Model file for the job. Use its own axes, mm. Round coordinates to 2 decimals unless told otherwise and drop trailing zeros. Write each loop counter-clockwise with the first axis right and the second up, starting at its lowest first coordinate (ties: lowest second). Pieces come first, ordered by that corner, then holes. Notation, with made-up numbers: (-10, 7) - (36, 7) arc R30 ccw to (36, 32) - close; hole circle Ø4 at (-11.5, 71). An arc over 180 degrees is marked (long way). Answer as a JSON object with one key per item and string values. Group by question number.
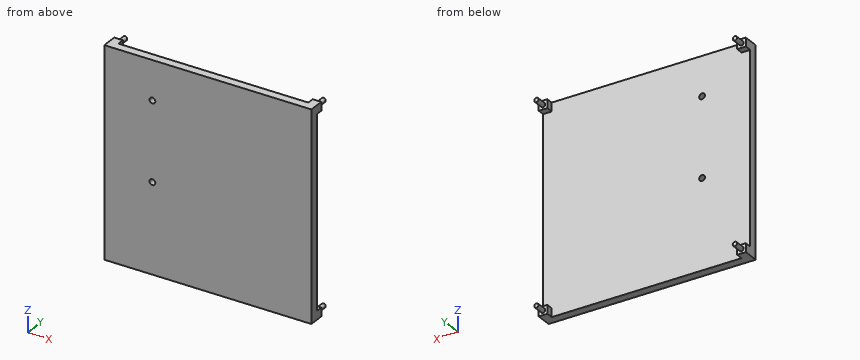
from build123d import *

# Parameters (mm, degrees)
STOCK_PLATE_BETA1_1_OUTLINE_W   = 152.4
STOCK_PLATE_BETA1_1_OUTLINE_H   = 152.4
STOCK_PLATE_BETA1_1_OUTLINE_R   = 2.125
STOCK_PLATE_BETA1_1_DEPTH       = 6.35
STOCK_PLATE_BETA1_1_START       = 6.35
STOCK_PLATE_BETA1_1_2_OUTLINE_W = 6.35
STOCK_PLATE_BETA1_1_2_OUTLINE_H = 6.35
STOCK_PLATE_BETA1_1_2_DEPTH     = 5.08
SKETCH1_R                       = 1.5875
BOSS_EXTRUDE1_DEPTH             = 7.62


# Read off the part's stored shape, not the designer's step: Stock-plate_beta1-1
with BuildPart() as part:
    # Stock-plate_beta1-1 outline → Stock-plate_beta1-1 (new body)
    with BuildSketch(Plane(origin=(0, 0, 0), x_dir=(1, 0, 0), z_dir=(0, 1, 0))):
        with Locations((40.776583963, 45.362139437)):
            Rectangle(STOCK_PLATE_BETA1_1_OUTLINE_W, STOCK_PLATE_BETA1_1_OUTLINE_H)
        with Locations((0, -2.125)):
            Circle(STOCK_PLATE_BETA1_1_OUTLINE_R, mode=Mode.SUBTRACT)
        with Locations((0, 55.889)):
            Circle(STOCK_PLATE_BETA1_1_OUTLINE_R, mode=Mode.SUBTRACT)
    extrude(amount=STOCK_PLATE_BETA1_1_DEPTH)

    # Stock-plate_beta1-1 2 outline → Stock-plate_beta1-1 2 (add)
    with BuildSketch(Plane(origin=(0, 0, 0), x_dir=(1, 0, 0), z_dir=(0, 1, 0)).offset(STOCK_PLATE_BETA1_1_START)):
        with Locations((113.801583963, 118.387139437)):
            Rectangle(STOCK_PLATE_BETA1_1_2_OUTLINE_W, STOCK_PLATE_BETA1_1_2_OUTLINE_H)
        with Locations((-32.248416037, 118.387139437)):
            Rectangle(STOCK_PLATE_BETA1_1_2_OUTLINE_W, STOCK_PLATE_BETA1_1_2_OUTLINE_H)
        with Locations((113.801583963, -27.662860563)):
            Rectangle(STOCK_PLATE_BETA1_1_2_OUTLINE_W, STOCK_PLATE_BETA1_1_2_OUTLINE_H)
        with Locations((-32.248416037, -27.662860563)):
            Rectangle(STOCK_PLATE_BETA1_1_2_OUTLINE_W, STOCK_PLATE_BETA1_1_2_OUTLINE_H)
    extrude(amount=STOCK_PLATE_BETA1_1_2_DEPTH)

    # Sketch1 → Boss-Extrude1 (add)
    with BuildSketch(Plane(origin=(0, 11.43, 0), x_dir=(1, 0, 0), z_dir=(0, 1, 0))):
        with Locations(Location((-32.248416037, -27.662860563, 0), (0, 0, 90))):
            Circle(SKETCH1_R)
        with Locations(Location((-32.225272977, 118.387139437, 0), (0, 0, 90))):
            Circle(SKETCH1_R)
        with Locations(Location((113.801583963, 118.387139437, 0), (0, 0, 90))):
            Circle(SKETCH1_R)
        with Locations(Location((113.801583963, -27.662860563, 0), (0, 0, 90))):
            Circle(SKETCH1_R)
    extrude(amount=BOSS_EXTRUDE1_DEPTH)


solid = part.part
(1) Flat gauge pins, fed straight in: pin 1 (2 mm diameter, centred on x = 30.5, z = -26, fed in from -Y); pin 2 (5 mm diameter, centred on x = 26.5, z = -20.5, fed in from +Y). Where does each tip first touch, or does it go through?
(2) Slice it at C-C (z = -61.5). Write the cut outline in (x, y).
(3) Slice it at A-A (x = 0). Write the cut outline in (y, z), then the cut area to 3 significant figures.
(4) Slice it at B-B (y = 8.75). Write the cut outline in (x, z).
(5) Drill centre lines: line 1 (Z direction, x = 0, y = 4); line 2 (Y direction, x = 93.5, z = -76); line 3 (X direction, y = 3.25, z = 1). Where is each one in solid material? Low to high. Write a range as from..to.
Answer:
{
 "1": {"pin 1": "y = 0", "pin 2": "y = 6.35"},
 "2": {"outline": "(-35.42, 0) - (116.98, 0) - (116.98, 6.35) - (-35.42, 6.35) - close"},
 "3": {"outline": "(0, -121.56) - (6.35, -121.56) - (6.35, -58.01) - (0, -58.01) - close; (0, -53.76) - (6.35, -53.76) - (6.35, 0) - (0, 0) - close; (0, 4.25) - (6.35, 4.25) - (6.35, 30.84) - (0, 30.84) - close", "area": "914 mm²"},
 "4": {"outline": "(-35.42, -121.56) - (-29.07, -121.56) - (-29.07, -115.21) - (-35.42, -115.21) - close; (-35.42, 24.49) - (-29.07, 24.49) - (-29.07, 30.84) - (-35.42, 30.84) - close; (110.63, -121.56) - (116.98, -121.56) - (116.98, -115.21) - (110.63, -115.21) - close; (110.63, 24.49) - (116.98, 24.49) - (116.98, 30.84) - (110.63, 30.84) - close"},
 "5": {"line 1": "-121.56..-58.01, -53.76..0, 4.25..30.84", "line 2": "0..6.35", "line 3": "-35.42..-1.8, 1.8..116.98"}
}
